The listing builds one solid part. Answer for the finished solid, in the listing's coordinates (mm). A direction names the side the tool comes from. Give positions to 0.01 mm unless a question says otherwise; leave off trailing zeros. Loops run counter-clockwise (first coordinate to the right, second up) from the corner with the lowest first, then second, coordinate; pieces in that order, holes last. Notation, with made-up numbers: M 47.5,68.25 L 73.5,68.25 A11 cw 73.5,87.25 Z; hole C -12,13.5 d3. An arc over 180 degrees is marked long. Return JSON: item names as keys, results as strings.
from build123d import *

# Parameters (mm, degrees)
SKETCH1_W           = 100
SKETCH1_H           = 4
BOSS_EXTRUDE1_DEPTH = 3


with BuildPart() as part:
    # Sketch1 → Boss-Extrude1 (new body)
    with BuildSketch(Plane.XY):
        Polygon((104.8, 73), (78.6, 73), (78.6, 70), (52.4, 70), (52.4, 73), (26.2, 73), (26.2, 70), (3, 70), (3, 46.8), (0, 46.8), (0, 20.6), (3, 20.6), (3, 3), (26.2, 3), (26.2, 0), (52.4, 0), (52.4, 3), (78.6, 3), (78.6, 0), (104.8, 0), (104.8, 3), (128, 3), (128, 20.6), (131, 20.6), (131, 46.8), (128, 46.8), (128, 70), (104.8, 70), align=None)
        with Locations((66, 17)):
            Rectangle(SKETCH1_W, SKETCH1_H, mode=Mode.SUBTRACT)
        with Locations((66, 25)):
            Rectangle(SKETCH1_W, SKETCH1_H, mode=Mode.SUBTRACT)
        with Locations((66, 33)):
            Rectangle(SKETCH1_W, SKETCH1_H, mode=Mode.SUBTRACT)
        with Locations((66, 41)):
            Rectangle(SKETCH1_W, SKETCH1_H, mode=Mode.SUBTRACT)
        with Locations((65.921603012, 48.672040999)):
            Rectangle(SKETCH1_W, SKETCH1_H, mode=Mode.SUBTRACT)
        with Locations((65.787326392, 56.191531722)):
            Rectangle(SKETCH1_W, SKETCH1_H, mode=Mode.SUBTRACT)
    extrude(amount=BOSS_EXTRUDE1_DEPTH)


solid = part.part
(1) Determine the mould class of faces 5 (the flat face through (65, 50.672, 1)), 6 (the flat face through (15, 70, 1)), 7 (the flat face through (65, 27, 1)), 8 (the flat face through (3, 59, 1)) for opening direction X: released by +X, released by -X, zero draft, split by the parting line, or undercut.
Values follow:
{"face 5": "undercut", "face 6": "zero draft", "face 7": "undercut", "face 8": "released by -X"}
(2) The part is cut by section A-A (x = 109). Determine the outline of the cut face in (y, z).
Values follow:
{"outline": "M 3,0 L 15,0 L 15,3 L 3,3 Z; M 19,0 L 23,0 L 23,3 L 19,3 Z; M 27,0 L 31,0 L 31,3 L 27,3 Z; M 35,0 L 39,0 L 39,3 L 35,3 Z; M 43,0 L 46.67,0 L 46.67,3 L 43,3 Z; M 50.67,0 L 54.19,0 L 54.19,3 L 50.67,3 Z; M 58.19,0 L 70,0 L 70,3 L 58.19,3 Z"}
(3) The part is cut by section C-C (z = 1). Give the number of separate pieces and of enclosed holes in the cut face, and give its area (3 significant figures).
Values follow:
{"separate pieces": "1", "enclosed holes": "6", "area": "6,450 mm²"}
(4) A tool of negligible diameter and unlimited length cuts with its end or side. For faces 1 (the flat face through (78.6, 2, 1)), 2 (the flat face through (130, 46.8, 1)), 3 (the flat face through (116, 25, 1)), 4 (the flat face through (1, 20.6, 1)), from which of +Z, -Z, +X, -X, +Y, -Y can it reach the whole face along a straight path? Write none if from no direction.
Values follow:
{"face 1": "+Z, -Z, -Y", "face 2": "+Z, -Z, +X, +Y", "face 3": "+Z, -Z", "face 4": "+Z, -Z, -X, -Y"}
(5) Given pin 1 (0.9 mm diameter, centred on y = 56, z = 1.5, fed in from -X); pin 2 (0.9 mm diameter, centred on y = 33, z = 2, fed in from -X); pin 3 (0.9 mm diameter, centred on y = 1, z = 2, fed in from +X); pin 4 (0.9 mm diameter, centred on x = 130, z = 1.5, fed in from +Y), each flat-ended and moving along its own axis, determine where each tip first touches the part or whether it passes through.
Values follow:
{"pin 1": "x = 3", "pin 2": "x = 0", "pin 3": "x = 104.8", "pin 4": "y = 46.8"}
(6) The part is cut by section D-D (x = 8). Determine the outline of the cut face in (y, z), and give its area (3 significant figures).
Values follow:
{"outline": "M 3,0 L 70,0 L 70,3 L 3,3 Z", "area": "201 mm²"}
(7) Straight lines are drawn through the part: line 1 along X through (y, z) = (18.5, 1.95); line 2 along X through (y, z) = (56.5, 1.45); line 3 along Y through (x, z) = (12, 0.8). For each, find the intervals that lie inside material, in ascending order.
Values follow:
{"line 1": "3 to 16, 116 to 128", "line 2": "3 to 15.79, 115.79 to 128", "line 3": "3 to 70"}
(8) The part is cut by section B-B (x = 35.5). Determine the outline of the cut face in (y, z).
Values follow:
{"outline": "M 0,0 L 15,0 L 15,3 L 0,3 Z; M 19,0 L 23,0 L 23,3 L 19,3 Z; M 27,0 L 31,0 L 31,3 L 27,3 Z; M 35,0 L 39,0 L 39,3 L 35,3 Z; M 43,0 L 46.67,0 L 46.67,3 L 43,3 Z; M 50.67,0 L 54.19,0 L 54.19,3 L 50.67,3 Z; M 58.19,0 L 73,0 L 73,3 L 58.19,3 Z"}
